The model under review builds one solid part; all positions refer to its coordinate system, in mm. Face numbers are marked on the shaded views. A direction names the side the tool comes from. Give positions to 0.01 mm unless a question says otherwise; leave off trailing zeros. Order: outer loops, then holes, each group sorted by start corner. A loop starts at its lowest first (then second) coordinate and runs counter-clockwise, first axis right, second up. Notation, with made-up numbers: (14.5, 41.5) - (61.5, 41.5) arc R7 ccw to (61.5, 54.5) - close; hole circle Ø5 at (11, 75). An arc over 180 degrees is marked (long way). Answer as CSV lines item,"result". Start each with the question number.
from build123d import *

# Parameters (mm, degrees)
F0_W      = 70
F0_H      = 70
F1_DEPTH  = 5
F2_W      = 60
F2_H      = 60
F3_DEPTH  = 26
F4_R      = 2.2
F5_DEPTH  = 10
F6_DEPTH  = 31.001
F7_DEPTH  = 2
F8_R      = 1.6
F9_DEPTH  = 70.001
F10_START = -7
F10_DEPTH = 18
F11_R     = 3
F12_SIZE  = 1


with BuildPart() as f1:
    # F0 (on Top) → F1 (new body)
    with BuildSketch(Plane.XY):
        Rectangle(F0_W, F0_H)
    extrude(amount=F1_DEPTH)

    # F2 (on face) → F3 (join)
    with BuildSketch(Plane.XY.offset(5)):
        with Locations((0, 5)):
            Rectangle(F2_W, F2_H)
    extrude(amount=F3_DEPTH)

    # F4 (on face) → F5 (cut)
    with BuildSketch(Plane.XY.offset(31)):
        with Locations((-23.5, -18.5)):
            Circle(F4_R)
        with Locations((-23.5, 28.5)):
            Circle(F4_R)
        with Locations((23.5, 28.5)):
            Circle(F4_R)
        with Locations((23.5, -18.5)):
            Circle(F4_R)
    extrude(amount=-F5_DEPTH, mode=Mode.SUBTRACT)

    # F4 (on face) → F6 (cut, through all)
    with BuildSketch(Plane.XY.offset(31)):
        with BuildLine():
            ThreePointArc((-15, 5), (0, -10), (15, 5))
            ThreePointArc((15, 5), (0, 20), (-15, 5))
        make_face()
        with BuildLine():
            Line((15, -6.9047259523), (15, 5))
            ThreePointArc((15, 5), (0, -10), (-15, 5))
            Line((-15, 5), (-15, -6.9047259523))
            ThreePointArc((-15, -6.9047259523), (0, -14.15), (15, -6.9047259523))
        make_face()
        with BuildLine():
            Line((15, -25), (15, -6.9047259523))
            ThreePointArc((15, -6.9047259523), (0, -14.15), (-15, -6.9047259523))
            Line((-15, -6.9047259523), (-15, -25))
            Line((-15, -25), (15, -25))
        make_face()
    extrude(amount=-F6_DEPTH, mode=Mode.SUBTRACT)

    # F4 (on face) → F7 (cut)
    with BuildSketch(Plane.XY.offset(31)):
        with BuildLine():
            ThreePointArc((-15, 5), (0, 20), (15, 5))
            Line((15, 5), (15, -6.9047259523))
            ThreePointArc((15, -6.9047259523), (18.0827611277, -1.3036695662), (19.15, 5))
            ThreePointArc((19.15, 5), (-6.3036695662, 23.0827611277), (-15, -6.9047259523))
            Line((-15, -6.9047259523), (-15, 5))
        make_face()
    extrude(amount=-F7_DEPTH, mode=Mode.SUBTRACT)

    # F8 (on face) → F9 (cut, through all)
    with BuildSketch(Plane(origin=(0, 35, 0), x_dir=(-1, 0, 0), z_dir=(0, 1, 0))):
        with Locations((0, 16)):
            Circle(F8_R)
    extrude(amount=-F9_DEPTH, mode=Mode.SUBTRACT)

    # F8 (on face) → F10 (cut)
    with BuildSketch(Plane(origin=(0, 35, 0), x_dir=(-1, 0, 0), z_dir=(0, 1, 0)).offset(F10_START)):
        Polygon((3.1754264805, 16), (1.5877132403, 18.75), (-1.5877132403, 18.75), (-3.1754264805, 16), (-1.5877132403, 13.25), (1.5877132403, 13.25), align=None)
        with Locations((0, 16)):
            Circle(F8_R, mode=Mode.SUBTRACT)
    extrude(amount=-F10_DEPTH, mode=Mode.SUBTRACT)

    # F11
    f11_edges = [f1.edges().sort_by_distance(p)[0] for p in [
        (30, -25, 18),
        (-30, -25, 18),
        (30, 35, 18),
        (-30, 35, 18),
        (-15, -25, 18),
        (15, -25, 18),
    ]]
    fillet(f11_edges, radius=F11_R)

    # F12
    f12_edges = [f1.edges().sort_by_distance(p)[0] for p in [
        (-35, 0, 5),
        (0, -35, 5),
        (35, 0, 5),
        (32.5, 35, 5),
        (-32.5, 35, 5),
        (35, -35, 2.5),
        (-35, -35, 2.5),
        (-35, 35, 2.5),
        (35, 35, 2.5),
    ]]
    chamfer(f12_edges, length=F12_SIZE)


solid = f1.part
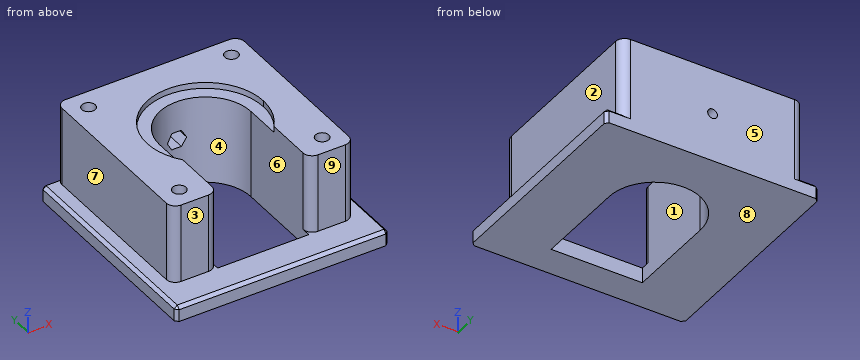
Item 1: For line 1 along Y through (x, z) = (23.5, 24); line 2 along X through (y, z) = (-6, 25); line 3 along X through (y, z) = (28, 23), list the stretches that pass through material, from the lowest coordinate up.
Item 2: Machinability: for the marked faces 5, 6, 7, 8 and 9, which of the approach directions +Z, -Z, +X, -X, +Y, -Y give a long, thin tool a straight path to every point of the face, cutting with its end or side? Answer none if there is none.
Item 3: Take a section at B-B on y = -18.5. Write out the cut boundary in (x, z).
Item 4: Take a section at D-D on x = 12. Write out the cut boundary in (y, z).
Item 5: Clearance check with flat-ended pins moving along their axes: pin 1 (2 mm diameter, centred on x = 12.5, y = 9.5, fed in from +Z); pin 2 (3 mm diameter, centred on x = 14.5, z = 18, fed in from -Y); pin 3 (1.5 mm diameter, centred on x = 22.5, y = 13.5, fed in from -Z); pin 4 (5 mm diameter, centred on x = 0, z = 16, fed in from -Y). State where each tip first meets the part, or that it passes through.
Item 6: Take a section at A-A on x = 0. Write out the cut boundary in (y, z).
Item 7: Take a section at C-C on z = 3. Write out the cut boundary in (x, y), and give its area (3 significant figures).
Item 8: Mouldability with a two-part tool opening along X and no side actions: class the marked faces 1, 2, 3 and 4 as released by +X, released by -X, zero draft, split by the parting line, or undercut.
Data:
1,line 1,"y = -25 to -20.7, -16.3 to 26.3, 30.7 to 35"
1,line 2,"x = -30 to -15, 15 to 30"
1,line 3,"x = -30 to -25.64, -21.36 to 21.36, 25.64 to 30"
2,face 5,"+Z, -Z, +X, -X, +Y"
2,face 6,"+Z, -Z"
2,face 7,"+Z, -X, +Y, -Y"
2,face 8,"-Z, +X, -X, +Y, -Y"
2,face 9,"+Z, +X, -X, -Y"
3,outline,"(-35, 0) - (-15, 0) - (-15, 31) - (-21.3, 31) - (-21.3, 21) - (-25.7, 21) - (-25.7, 31) - (-30, 31) - (-30, 5) - (-34, 5) - (-35, 4) - close; (15, 0) - (35, 0) - (35, 4) - (34, 5) - (30, 5) - (30, 31) - (25.7, 31) - (25.7, 21) - (21.3, 21) - (21.3, 31) - (15, 31) - close"
4,outline,"(-35, 0) - (-25, 0) - (-25, 5) - (-34, 5) - (-35, 4) - close; (14, 0) - (35, 0) - (35, 31) - (19.92, 31) - (19.92, 29) - (14, 29) - close"
5,pin 1,"passes through"
5,pin 2,"stops at y = -24.24"
5,pin 3,"stops at z = 0"
5,pin 4,"stops at y = 28"
6,outline,"(-35, 0) - (-25, 0) - (-25, 5) - (-34, 5) - (-35, 4) - close; (20, 0) - (35, 0) - (35, 14.4) - (28, 14.4) - (28, 13.25) - (20, 13.25) - close; (20, 18.75) - (28, 18.75) - (28, 17.6) - (35, 17.6) - (35, 31) - (24.15, 31) - (24.15, 29) - (20, 29) - close"
7,outline,"(-35, -34) - (-34, -35) - (34, -35) - (35, -34) - (35, 34) - (34, 35) - (-34, 35) - (-35, 34) - close; hole (-15, -25) - (15, -25) - (15, 5) arc R15 ccw to (-15, 5) - close"
7,area,"3,640 mm^2"
8,face 1,"undercut"
8,face 2,"released by +X"
8,face 3,"zero draft"
8,face 4,"undercut"
